from build123d import *

# Parameters (mm, degrees)
CYLINDER100_R     = 1.7
CYLINDER100_DEPTH = 12
CYLINDER099_R     = 3
CYLINDER099_DEPTH = 3
CYLINDER098_R     = 3.75
CYLINDER098_DEPTH = 10
CYLINDER097_R     = 5.5
CYLINDER097_DEPTH = 2
CUT051_ROLL_ANGLE = -90


with BuildPart() as obj1:
    # Cylinder100 → Cylinder100 (new body)
    with BuildSketch(Plane.XY):
        Circle(CYLINDER100_R)
    extrude(amount=CYLINDER100_DEPTH)


with BuildPart() as obj2:
    # Cylinder099 → Cylinder099 (new body)
    with BuildSketch(Plane.XY):
        Circle(CYLINDER099_R)
    extrude(amount=CYLINDER099_DEPTH)


with BuildPart() as obj3:
    # Cone007 → Cone007 (revolve)
    with BuildSketch(Plane(origin=(0, 0, 3), x_dir=(1, 0, 0), z_dir=(0, -1, 0))):
        Polygon((0, 0), (3, 0), (1.7, 1.3), (0, 1.3), align=None)
    revolve(axis=Axis((0, 0, 3), (0, 0, 1)))


with BuildPart() as cylinder117:
    # Cylinder098 → Cylinder098 (new body)
    with BuildSketch(Plane.XY.offset(2)):
        Circle(CYLINDER098_R)
    extrude(amount=CYLINDER098_DEPTH)


with BuildPart() as springguide:
    # Cylinder097 → Cylinder097 (new body)
    with BuildSketch(Plane.XY):
        Circle(CYLINDER097_R)
    extrude(amount=CYLINDER097_DEPTH)

    # Fusion004: union Cylinder117
    add(cylinder117.part)

    # Cut049: cut obj3
    add(obj3.part, mode=Mode.SUBTRACT)

    # Cut050: cut obj2
    add(obj2.part, mode=Mode.SUBTRACT)

    # Cut051: cut obj1
    add(obj1.part, mode=Mode.SUBTRACT)


with BuildPart() as springguide_1:
    # Cut051 roll: moved
    add(springguide.part.rotate(Axis((0, 0, 0), (1, 0, 0)), CUT051_ROLL_ANGLE))


with BuildPart() as springguide_2:
    # Cut051 placement: moved
    add(springguide_1.part.moved(Location((19, -70, 10))))


solid = springguide_2.part
Check sheet for the modelled part. Datum: model origin and axes. Units: mm. Coordinates: 2 decimals unless noted, no trailing zeros. Write each loop counter-clockwise with the first axis right and the second up, starting at its lowest first coordinate (ties: lowest second). Pieces come first, ordered by that corner, then holes. Notation, with made-up numbers: M 39.5,-39.75 L 74.5,-39.75 A20 ccw 74.5,-26.75 Z; hole C 78,38.5 d5. An arc over 180 degrees is marked long. Answer as CSV lines item,"result".
Q1. Material ranges on probe 1 along X at (y, z) = (-69.2, 10); probe 2 along X at (y, z) = (-64, 10); probe 3 along Z at (x, y) = (19, -69.15), recorded low to high. Write a range as from..to.
Check result:
probe 1,"13.5..16, 22..24.5"
probe 2,"15.25..17.3, 20.7..22.75"
probe 3,"4.5..7, 13..15.5"
Q2. Cross-section at D-D (z = 13.25). Record the boundary of the cut face in (x, y), then the cut area to 3 significant figures.
Check result:
outline,"M 14.56,-70 L 23.44,-70 L 23.44,-68 L 20.87,-68 L 20.87,-58 L 17.13,-58 L 17.13,-68 L 14.56,-68 Z"
area,"55.2 mm^2"
Q3. Go/stop test with flat-tipped pins: pin 1 (3 mm diameter, centred on y = -61.5, z = 7, fed in from +X); pin 2 (3 mm diameter, centred on x = 21, y = -62.5, fed in from +Z); pin 3 (4 mm diameter, centred on y = -68.5, z = 13, fed in from +X). Record where each tip stops, or that it passes through.
Check result:
pin 1,"x = 22.44"
pin 2,"z = 13.72"
pin 3,"x = 24.41"
Q4. Cross-section at B-B (z = 10). Record the boundary of the cut face in (x, y).
Check result:
outline,"M 13.5,-70 L 16,-70 L 16,-67 L 17.3,-65.7 L 17.3,-58 L 15.25,-58 L 15.25,-68 L 13.5,-68 Z; M 20.7,-65.7 L 22,-67 L 22,-70 L 24.5,-70 L 24.5,-68 L 22.75,-68 L 22.75,-58 L 20.7,-58 Z"
Q5. Cross-section at C-C (y = -63.5). Record the boundary of the cut face in (x, z), then the cut area to 3 significant figures.
Check result:
outline,"C 19,10 d7.5; hole C 19,10 d3.4"
area,"35.1 mm^2"
Q6. Cross-section at A-A (x = 19). Record the boundary of the cut face in (y, z).
Check result:
outline,"M -70,4.5 L -68,4.5 L -68,6.25 L -58,6.25 L -58,8.3 L -65.7,8.3 L -67,7 L -70,7 Z; M -70,13 L -67,13 L -65.7,11.7 L -58,11.7 L -58,13.75 L -68,13.75 L -68,15.5 L -70,15.5 Z"
Q7. Mould release check, pull along X, two halves, no side actions. Record for faces 1 (the face through (16.236, -63.07, 7.466)), 2 (the face through (19, -66, 8)), 3 (the face through (16, -69, 10)), 4 (the face through (23, -68, 11)): released by +X, released by -X, zero draft, split by the parting line, or undercut.
Check result:
face 1,"split by the parting line"
face 2,"undercut"
face 3,"undercut"
face 4,"zero draft"
